Drawing for the job (mm, zero at the part's lowest x, y, z). A direction names the side the tool comes from. Round coordinates to 2 decimals unless told otherwise and drop trailing zeros. Loops run counter-clockwise (first coordinate to the right, second up) from the corner with the lowest first, then second, coordinate; pieces in that order, holes last.
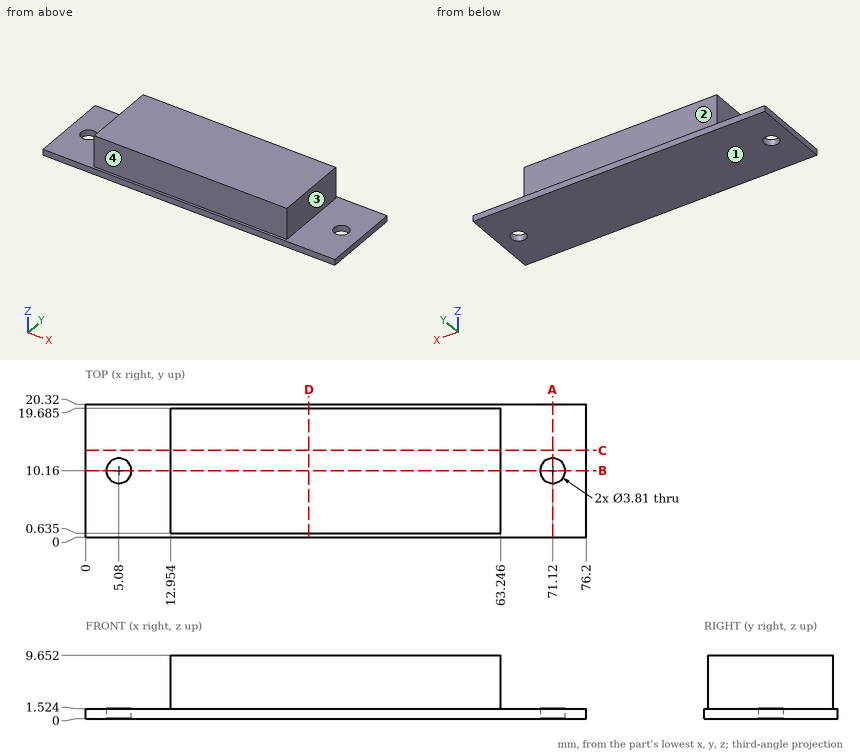
Q1. Slice it at C-C on y = 13.25. Give the cut face in (x, z), plus the area to 3 significant figures.
Q2. Slice it at B-B on y = 10.16. Give the cut face in (x, z) (3 decimals), plus the area to 3 significant figures.
Q3. Tool access for the marked faces 1, 2, 3 and 4: list every direction of +Z, -Z, +X, -X, +Y, -Y with a clear straight run to the whole face (end or side of a thin tool).
Q4. Flat gauge pins, fed straight in: P1, Ø1.5, axis at y = 14, z = 5, coming from the +X side; P2, Ø2, axis at x = 31, y = 17, coming from the -Z side; P3, Ø3.5, axis at x = 71.12, y = 10.16, coming from the +Z side; P4, Ø2.5, axis at x = 50.5, z = 7, coming from the +Y side (3 decimals). Where does each tip first touch, or does it go through?
Q5. Slice it at A-A on x = 71.12. Give the cut face in (y, z) (3 decimals), plus the area to 3 significant figures.
Q6. Probe line 1 (Y direction, x = 5.08, z = 1.1) (3 decimals); line 2 (Y direction, x = 16.5, z = 6.75) (3 decimals); line 3 (X direction, y = 12.75, z = 8.75). List the from-to ranges inside material, lowest first.
Q7. Slice it at D-D on x = 34. Give the cut face in (y, z) (3 decimals), plus the area to 3 significant figures.
Reply:
1. outline: (0, 0) - (76.2, 0) - (76.2, 1.52) - (63.25, 1.52) - (63.25, 9.65) - (12.95, 9.65) - (12.95, 1.52) - (0, 1.52) - close
1. area: 525 mm2
2. outline: (0, 0) - (3.175, 0) - (3.175, 1.524) - (0, 1.524) - close; (6.985, 0) - (69.215, 0) - (69.215, 1.524) - (63.246, 1.524) - (63.246, 9.652) - (12.954, 9.652) - (12.954, 1.524) - (6.985, 1.524) - close; (73.025, 0) - (76.2, 0) - (76.2, 1.524) - (73.025, 1.524) - close
2. area: 513 mm2
3. face 1: -Z, +X, -X, +Y, -Y
3. face 2: +Z, +X, -X, +Y
3. face 3: +Z, +X, +Y, -Y
3. face 4: +Z, +X, -X, -Y
4. P1: stops at x = 63.25
4. P2: stops at z = 0
4. P3: passes through
4. P4: stops at y = 19.685
5. outline: (0, 0) - (8.255, 0) - (8.255, 1.524) - (0, 1.524) - close; (12.065, 0) - (20.32, 0) - (20.32, 1.524) - (12.065, 1.524) - close
5. area: 25.2 mm2
6. line 1: y = 0 to 8.255, 12.065 to 20.32
6. line 2: y = 0.635 to 19.685
6. line 3: x = 12.95 to 63.25
7. outline: (0, 0) - (20.32, 0) - (20.32, 1.524) - (19.685, 1.524) - (19.685, 9.652) - (0.635, 9.652) - (0.635, 1.524) - (0, 1.524) - close
7. area: 186 mm2
